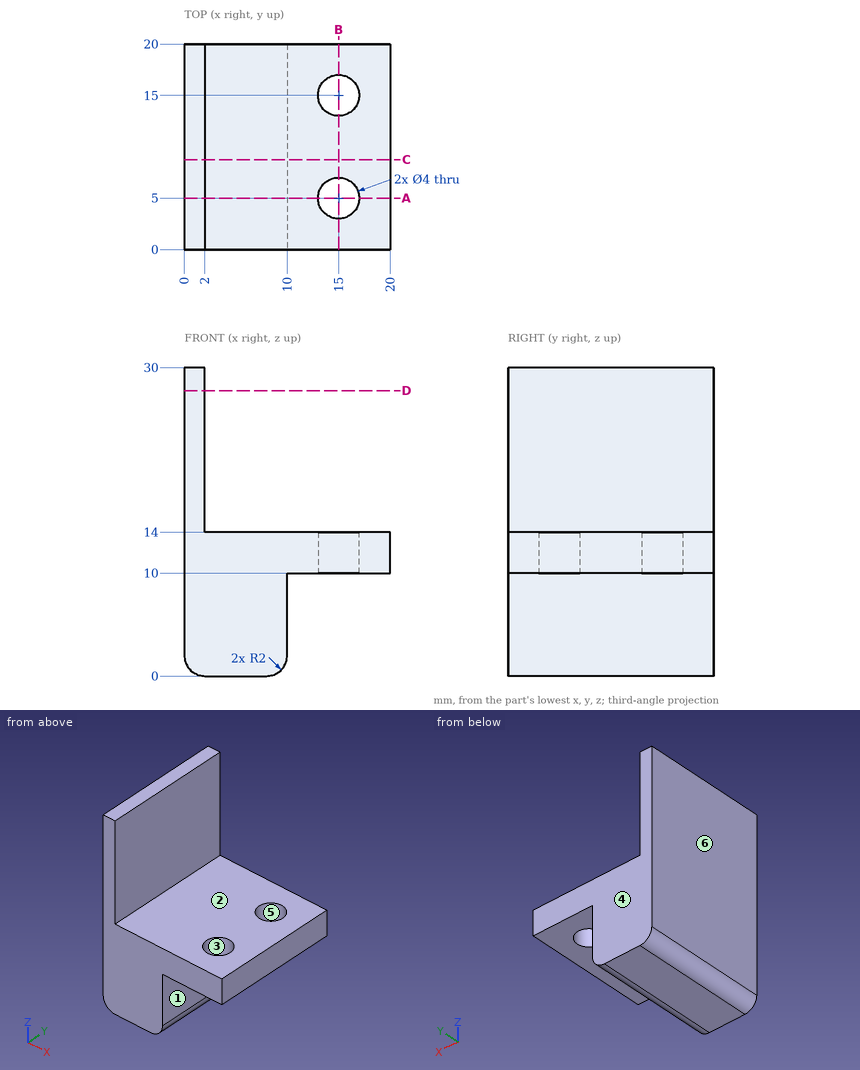
Verification items for this drawing (mm, ordinates from the low corner). A direction names the side the tool comes from. Round coordinates to 2 decimals unless told otherwise and drop trailing zeros. Write each loop counter-clockwise with the first axis right and the second up, starting at its lowest first coordinate (ties: lowest second). Pieces come first, ordered by that corner, then holes. Notation, with made-up numbers: (-20.75, -32) - (31.25, -32) arc R10 ccw to (31.25, -20) - close; hole circle Ø8 at (73, 40.25). An arc over 180 degrees is marked (long way). Answer as a JSON object with one key per item and string values. Group by question number.
Q1. Thickness scan on line 1 (Y direction, x = 15, z = 12.5); line 2 (X direction, y = 15, z = 10.8); line 3 (X direction, y = 10.25, z = 7.75). Record the ranges inside material, lowest first.
Q2. Mould release check, pull along Y, two halves, no side actions. Record for the marked faces 4, 5 and 6: released by +Y, released by -Y, zero draft, split by the parting line, or undercut.
Q3. Section check C-C, the plane y = 8.75. Enter the section's corners in (x, z).
Q4. Section check D-D, the plane z = 27.75. Enter the section's corners in (x, y).
Q5. Tool access check on the marked faces 1, 2 and 3. Record the directions out of +Z, -Z, +X, -X, +Y, -Y that give a thin tool (end or side, any length) a straight path to the whole face; none if there is none.
Q6. Section check A-A, the plane y = 5. Enter the section's corners in (x, z), plus the area to 3 significant figures.
Q7. Section check B-B, the plane x = 15. Enter the section's corners in (y, z), plus the area to 3 significant figures.
Q8. Go/stop test with flat-tipped pins: pin 1 Ø4.5 at (x, y) = (15, 15) entering from +Z; pin 2 Ø3 at (x, y) = (15.5, 11.5) entering from -Z; pin 3 Ø4 at (y, z) = (13, 6.5) entering from +X. Record where each tip stops, or that it passes through.
Found:
{
 "1": {"line 1": "y = 0 to 3, 7 to 13, 17 to 20", "line 2": "x = 0 to 13, 17 to 20", "line 3": "x = 0 to 10"},
 "2": {"face 4": "released by +Y", "face 5": "undercut", "face 6": "zero draft"},
 "3": {"outline": "(0, 2) arc R2 ccw to (2, 0) - (8, 0) arc R2 ccw to (10, 2) - (10, 10) - (20, 10) - (20, 14) - (2, 14) - (2, 30) - (0, 30) - close"},
 "4": {"outline": "(0, 0) - (2, 0) - (2, 20) - (0, 20) - close"},
 "5": {"face 1": "-Z, +X, +Y, -Y", "face 2": "+Z, +X, +Y, -Y", "face 3": "+Z, -Z"},
 "6": {"outline": "(0, 2) arc R2 ccw to (2, 0) - (8, 0) arc R2 ccw to (10, 2) - (10, 10) - (13, 10) - (13, 14) - (2, 14) - (2, 30) - (0, 30) - close; (17, 10) - (20, 10) - (20, 14) - (17, 14) - close", "area": "194 mm^2"},
 "7": {"outline": "(0, 10) - (3, 10) - (3, 14) - (0, 14) - close; (7, 10) - (13, 10) - (13, 14) - (7, 14) - close; (17, 10) - (20, 10) - (20, 14) - (17, 14) - close", "area": "48.0 mm^2"},
 "8": {"pin 1": "stops at z = 14", "pin 2": "stops at z = 10", "pin 3": "stops at x = 10"}
}
